Geometry check sheet. Reference: the model listing, model coordinates, mm. Face numbers are marked on the shaded views. A direction names the side the tool comes from. Give positions to 0.01 mm unless a question says otherwise; leave off trailing zeros. Write each loop counter-clockwise with the first axis right and the second up, starting at its lowest first coordinate (ties: lowest second). Pieces come first, ordered by that corner, then holes. Notation, with made-up numbers: M 77,-10.75 L 104,-10.75 A23 cw 104,16.25 Z; hole C 86,38 d1. An arc over 180 degrees is marked long. One line per item, written item: value. Start each with the question number.
1. Cross-section at A-A on y = 15.5. Record the cut outline in (x, z).
2. Gauge pin test, flat ends, axial feed: pin 1 (2.5 mm diameter, centred on x = -20.35, y = 6.17, fed in from -Z); pin 2 (10 mm diameter, centred on y = 17, z = -4.5, fed in from -X); pin 3 (5 mm diameter, centred on x = 9, z = -6, fed in from -Y). Record the tip position at first contact, or that the pin passes through.
3. Cross-section at B-B on z = -9.5. Record the cut outline in (x, y), then the cut area to 3 significant figures.
4. Tool access check on the marked faces 1, 2, 3 and 4. Record the directions out of +Z, -Z, +X, -X, +Y, -Y that give a thin tool (end or side, any length) a straight path to the whole face; none if there is none.
5. Cross-section at C-C on x = -48. Record the cut outline in (y, z), then the cut area to 3 significant figures.
6. Cross-section at D-D on y = -18.5. Record the cut outline in (x, z), then the cut area to 3 significant figures.
7. Scan lines: line 1 (Y direction, x = -53.75, z = 1.1); line 2 (Y direction, x = 23.5, z = 1); line 3 (X direction, y = 26, z = -9.5). Record each from-to range of solid material in increasing order.
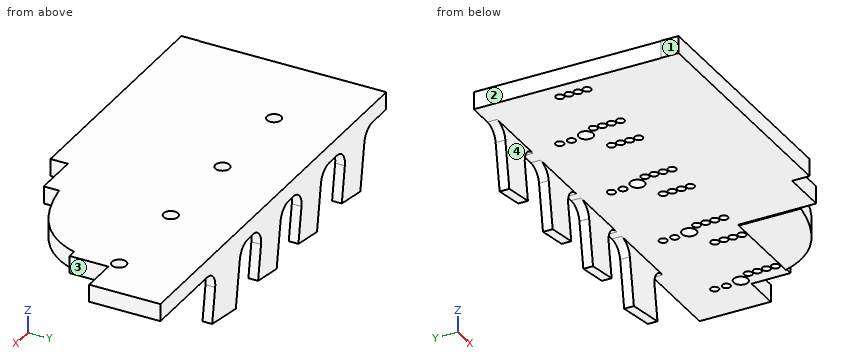
from build123d import *

# Parameters (mm, degrees)
SKETCH1_W           = 24.7
SKETCH1_H           = 21
SKETCH1_R           = 1.05
SKETCH1_R_2         = 1.85000003
SKETCH1_R_3         = 1.050000015
BOSS_EXTRUDE1_DEPTH = 2
LPATTERN1_COUNT     = 4
LPATTERN1_PITCH     = 24.7
SKETCH3_W           = 98.8
SKETCH3_H           = 21
SKETCH3_R           = 1.85000003
BOSS_EXTRUDE2_DEPTH = 2.5
SKETCH4_W           = 98.8
SKETCH4_H           = 4.5
BOSS_EXTRUDE3_DEPTH = 7.36771
SKETCH6_W           = 4.5
SKETCH6_H           = 18.36771
BOSS_EXTRUDE4_DEPTH = 9.198019
SKETCH7_W           = 74.1
SKETCH7_H           = 4.5
BOSS_EXTRUDE5_DEPTH = 20
SKETCH8_W           = 53.178454151
SKETCH8_H           = 4.5
BOSS_EXTRUDE6_DEPTH = 4.5
BOSS_EXTRUDE7_DEPTH = 4.75
BOSS_EXTRUDE8_DEPTH = 2.5
SKETCH14_W          = 4.5
SKETCH14_H          = 4.5
BOSS_EXTRUDE9_DEPTH = 9.5
FILLET1_R           = 4


with BuildPart() as part:
    # Sketch1 → Boss-Extrude1 (new body)
    with BuildSketch(Plane.XY):
        with Locations((12.35, 10.5)):
            Rectangle(SKETCH1_W, SKETCH1_H)
        with Locations((22.850000164, 18.500000119)):
            Circle(SKETCH1_R, mode=Mode.SUBTRACT)
        with Locations((22.850000164, 15.500000119)):
            Circle(SKETCH1_R, mode=Mode.SUBTRACT)
        with Locations((22.350000149, 11.500000015)):
            Circle(SKETCH1_R_2, mode=Mode.SUBTRACT)
        with Locations((20.350000119, 8.49999997)):
            Circle(SKETCH1_R_3, mode=Mode.SUBTRACT)
        with Locations((20.350000119, 6.166666637)):
            Circle(SKETCH1_R_3, mode=Mode.SUBTRACT)
        with Locations((20.350000119, 3.833333304)):
            Circle(SKETCH1_R_3, mode=Mode.SUBTRACT)
        with Locations((20.350000119, 1.49999997)):
            Circle(SKETCH1_R_3, mode=Mode.SUBTRACT)
        with Locations((4.349999881, 8.49999997)):
            Circle(SKETCH1_R_3, mode=Mode.SUBTRACT)
        with Locations((4.349999881, 6.166666637)):
            Circle(SKETCH1_R_3, mode=Mode.SUBTRACT)
        with Locations((4.349999881, 3.833333304)):
            Circle(SKETCH1_R_3, mode=Mode.SUBTRACT)
        with Locations((4.349999881, 1.49999997)):
            Circle(SKETCH1_R_3, mode=Mode.SUBTRACT)
    boss_extrude1 = extrude(amount=BOSS_EXTRUDE1_DEPTH)

    # LPattern1: Boss-Extrude1 ×4
    with Locations(*[(-i * LPATTERN1_PITCH, 0, 0) for i in range(1, LPATTERN1_COUNT)]):
        add(boss_extrude1)

    # Sketch3 → Boss-Extrude2 (add)
    with BuildSketch(Plane.XY.offset(2)):
        with Locations((-24.7, 10.5)):
            Rectangle(SKETCH3_W, SKETCH3_H)
        with Locations((-51.749999851, 11.500000015)):
            Circle(SKETCH3_R, mode=Mode.SUBTRACT)
        with Locations((-27.049999851, 11.500000015)):
            Circle(SKETCH3_R, mode=Mode.SUBTRACT)
        with Locations((-2.349999851, 11.500000015)):
            Circle(SKETCH3_R, mode=Mode.SUBTRACT)
        with Locations((22.350000149, 11.500000015)):
            Circle(SKETCH3_R, mode=Mode.SUBTRACT)
    extrude(amount=BOSS_EXTRUDE2_DEPTH)

    # Sketch4 → Boss-Extrude3 (add)
    with BuildSketch(Plane(origin=(0, 21, 0), x_dir=(1, 0, 0), z_dir=(0, 1, 0))):
        with Locations((-24.7, -2.25)):
            Rectangle(SKETCH4_W, SKETCH4_H)
    extrude(amount=BOSS_EXTRUDE3_DEPTH)

    # Sketch6 → Boss-Extrude4 (add)
    with BuildSketch(Plane(origin=(24.7, 0, 0), x_dir=(0, 0, -1), z_dir=(1, 0, 0))):
        with Locations((-2.25, 19.183855)):
            Rectangle(SKETCH6_W, SKETCH6_H)
    extrude(amount=BOSS_EXTRUDE4_DEPTH)

    # Sketch7 → Boss-Extrude5 (add)
    with BuildSketch(Plane.XZ):
        with Locations((-37.05, 2.25)):
            Rectangle(SKETCH7_W, SKETCH7_H)
    extrude(amount=BOSS_EXTRUDE5_DEPTH)

    # Sketch8 → Boss-Extrude6 (add)
    with BuildSketch(Plane.XZ.offset(20)):
        with Locations((-38.117142498, 2.25)):
            Rectangle(SKETCH8_W, SKETCH8_H)
    extrude(amount=BOSS_EXTRUDE6_DEPTH)

    # Sketch9 → Boss-Extrude7 (add)
    with BuildSketch(Plane.XY.offset(4.5)):
        with BuildLine():
            Line((0, 0), (0, -16.059466978))
            add(Edge.make_bspline(
                [(0, -16.059466978), (18.484574141, -13.097711422), (22.548154032, 0)],
                knots=[0, 0, 0, 0.956663175, 0.956663175, 0.956663175], degree=2))
            Line((22.548154032, 0), (0, 0))
        make_face()
    extrude(amount=-BOSS_EXTRUDE7_DEPTH)

    # Sketch10 → Boss-Extrude8 (add)
    with BuildSketch(Plane(origin=(0, 28.36771, 0), x_dir=(1, 0, 0), z_dir=(0, 1, 0))):
        Polygon((-64.88730383, -4.5), (-61.722013793, 15.247935056), (-52.835443017, 13.823554539), (-55.051146044, 0), (-43.421268353, 0), (-40.991049642, 15.161896923), (-32.104478867, 13.737516406), (-34.306391305, 0), (-24.086432643, 0), (-21.693532902, 14.929067518), (-12.806962127, 13.504687001), (-15.036483854, -0.405081066), (-4.619230317, 0), (-2.161338866, 15.334544441), (9.14228964, 13.522746772), (6.974801469, 0), (6.974801469, -4.5), align=None)
    extrude(amount=-BOSS_EXTRUDE8_DEPTH)

    # Sketch14 → Boss-Extrude9 (add)
    with BuildSketch(Plane.ZY.offset(64.706369573)):
        with Locations((2.25, -22.25)):
            Rectangle(SKETCH14_W, SKETCH14_H)
    extrude(amount=BOSS_EXTRUDE9_DEPTH)

    # Fillet1
    fillet1_edges = [part.edges().sort_by_distance(p)[0] for p in [
        (6.974801469, 27.11771, 0),
        (-4.619230317, 27.11771, 0),
        (-14.971555594, 27.11771, 0),
        (-24.086432643, 27.11771, 0),
        (-34.306391305, 27.11771, 0),
        (-43.421268353, 27.11771, 0),
        (-55.051146044, 27.11771, 0),
        (-64.166023092, 27.11771, 0),
    ]]
    fillet(fillet1_edges, radius=FILLET1_R)


solid = part.part
Report:
1. outline: M -74.1,0 L -52.3,0 L -52.3,2 L -50.2,2 L -50.2,0 L -27.6,0 L -27.6,2 L -25.5,2 L -25.5,0 L -2.9,0 L -2.9,2 L -0.8,2 L -0.8,0 L 21.8,0 L 21.8,2 L 23.9,2 L 23.9,0 L 33.9,0 L 33.9,4.5 L -74.1,4.5 Z
2. pin 1: stops at z = 0
2. pin 2: stops at x = -74.1
2. pin 3: stops at y = 25.87
3. outline: M -62.64,25.87 L -53.53,25.87 L -53.53,28.37 L -62.64,28.37 Z; M -41.9,25.87 L -32.78,25.87 L -32.78,28.37 L -41.9,28.37 Z; M -22.56,25.87 L -13.45,25.87 L -13.45,28.37 L -22.56,28.37 Z; M -3.1,25.87 L 8.5,25.87 L 8.5,28.37 L -3.1,28.37 Z
3. area: 97.3 mm^2
4. face 1: +Z, -Z, -X, +Y, -Y
4. face 2: +Z, -Z, -X, +Y
4. face 3: +Z, -Z, +X, -Y
4. face 4: -Z, +X, -X, -Y
5. outline: M -24.5,0 L 28.37,0 L 28.37,4.5 L -24.5,4.5 Z
5. area: 238 mm^2
6. outline: M -74.1,0 L 0,0 L 0,4.5 L -74.1,4.5 Z
6. area: 333 mm^2
7. line 1: y = -24.5 to 0.45, 2.55 to 2.78, 4.88 to 5.12, 7.22 to 7.45, 9.55 to 28.37
7. line 2: y = 0 to 10.05, 12.95 to 14.68, 16.32 to 17.68, 19.32 to 28.37
7. line 3: x = -62.64 to -53.53, -41.9 to -32.78, -22.56 to -13.45, -3.1 to 8.5
